```python
from build123d import *

# Parameters (mm, degrees)
F1_DEPTH = 10
F2_R     = 2.4
F3_DEPTH = 3
F7_R     = 5.08
F8_R     = 1.27


# Not quite as in the source:
# - a pattern or mirror of a feature is missing from the dataset's text; its kind, count and spacing are read off the source's solid


with BuildPart() as f1:
    # F0 (on Front) → F1 (new body)
    with BuildSketch(Plane.XZ):
        with BuildLine():
            ThreePointArc((0, 8.89), (6.2861792847, 6.2861792847), (8.89, 0))
            Line((8.89, 0), (8.89, -8.255))
            Line((8.89, -8.255), (21.89, -8.255))
            Line((21.89, -8.255), (21.89, -5.255))
            Line((21.89, -5.255), (11.89, -5.255))
            Line((11.89, -5.255), (11.89, 0))
            ThreePointArc((11.89, 0), (8.4074996283, 8.4074996283), (0, 11.89))
            Line((0, 11.89), (-5.255, 11.89))
            Line((-5.255, 11.89), (-5.255, 21.89))
            Line((-5.255, 21.89), (-8.255, 21.89))
            Line((-8.255, 21.89), (-8.255, 8.89))
            Line((-8.255, 8.89), (0, 8.89))
        make_face()
    extrude(amount=F1_DEPTH)

    # F2 (on face) → F3 (cut, through all)
    with BuildSketch(Plane.XY.offset(-5.255)):
        with Locations((16.89, -5)):
            Circle(F2_R)
    f3 = extrude(amount=-F3_DEPTH, mode=Mode.SUBTRACT)

    # F3_copies: F3 across plane
    add(f3.mirror(Plane(origin=(0, 0, 0), x_dir=(-0.7071067812, 0, -0.7071067812), z_dir=(-0.7071067812, 0, 0.7071067812))), mode=Mode.SUBTRACT)

    # F7
    f7_edges = [f1.edges().sort_by_distance(p)[0] for p in [
        (-8.255, -5, 8.89),
        (8.89, -5, -8.255),
    ]]
    fillet(f7_edges, radius=F7_R)

    # F8
    f8_edges = [f1.edges().sort_by_distance(p)[0] for p in [
        (-5.255, -5, 11.89),
        (11.89, -5, -5.255),
    ]]
    fillet(f8_edges, radius=F8_R)


solid = f1.part
```
Verification items for the finished model (mm, model axes). A direction names the side the tool comes from. Give positions to 0.01 mm unless a question says otherwise; leave off trailing zeros. Loops run counter-clockwise (first coordinate to the right, second up) from the corner with the lowest first, then second, coordinate; pieces in that order, holes last. Notation, with made-up numbers: M 40.25,71 L 48.25,71 A28 cw 48.25,107 Z; hole C -9.5,58 d4. An arc over 180 degrees is marked long. Return JSON: item names as keys, results as strings.
1) Section check D-D, the plane y = -1.5. Enter the section's corners in (x, z) (3 decimals), and give its area (3 significant figures).
Findings:
{"outline": "M -8.255,13.97 A5.08 ccw -3.175,8.89 L 0,8.89 A8.89 cw 8.89,0 L 8.89,-3.175 A5.08 ccw 13.97,-8.255 L 21.89,-8.255 L 21.89,-5.255 L 13.16,-5.255 A1.27 cw 11.89,-3.985 L 11.89,0 A11.89 ccw 0,11.89 L -3.985,11.89 A1.27 cw -5.255,13.16 L -5.255,21.89 L -8.255,21.89 Z", "area": "148 mm2"}
2) Mould release check, pull along Y, two halves, no side actions. Record for faces 1 (the flat face through (6, 0, 7)), 2 (the cylindrical face through (6.22, -4.93, 6.35)), 3 (the cylindrical face through (18.18, -2.976, -6.734)): released by +Y, released by -Y, zero draft, split by the parting line, or undercut.
Findings:
{"face 1": "released by +Y", "face 2": "zero draft", "face 3": "undercut"}
3) Section check A-A, the plane y = -5. Enter the section's corners in (x, z) (3 decimals), and give its area (3 significant figures).
Findings:
{"outline": "M -8.255,13.97 A5.08 ccw -3.175,8.89 L 0,8.89 A8.89 cw 8.89,0 L 8.89,-3.175 A5.08 ccw 13.97,-8.255 L 14.49,-8.255 L 14.49,-5.255 L 13.16,-5.255 A1.27 cw 11.89,-3.985 L 11.89,0 A11.89 ccw 0,11.89 L -3.985,11.89 A1.27 cw -5.255,13.16 L -5.255,14.49 L -8.255,14.49 Z; M -8.255,19.29 L -5.255,19.29 L -5.255,21.89 L -8.255,21.89 Z; M 19.29,-8.255 L 21.89,-8.255 L 21.89,-5.255 L 19.29,-5.255 Z", "area": "119 mm2"}
4) Section check C-C, the plane z = 16.89. Enter the section's corners in (x, y) (3 decimals), and give its area (3 significant figures).
Findings:
{"outline": "M -8.255,-10 L -5.255,-10 L -5.255,-7.4 L -8.255,-7.4 Z; M -8.255,-2.6 L -5.255,-2.6 L -5.255,0 L -8.255,0 Z", "area": "15.6 mm2"}
5) Material ranges on L1, parallel to X at y = -3, z = -1.5; L2, parallel to Z at x = 19.5, y = -8.25 (3 decimals), recorded low to high. Write a range as [from, to].
Findings:
{"L1": "x = [8.89, 11.89]", "L2": "z = [-8.255, -5.255]"}
6) Section check B-B, the plane x = 16.89. Enter the section's corners in (y, z) (3 decimals).
Findings:
{"outline": "M -10,-8.255 L -7.4,-8.255 L -7.4,-5.255 L -10,-5.255 Z; M -2.6,-8.255 L 0,-8.255 L 0,-5.255 L -2.6,-5.255 Z"}
7) Tool access check on faces 4 (the flat face through (8.89, -5, -2)), 5 (the flat face through (-8.255, -5, 20)), 6 (the flat face through (11.89, -5, -2)). Record the directions out of +Z, -Z, +X, -X, +Y, -Y that give a thin tool (end or side, any length) a straight path to the whole face; none if there is none.
Findings:
{"face 4": "-Z, -X, +Y, -Y", "face 5": "+Z, -Z, -X, +Y, -Y", "face 6": "+Z, +X, +Y, -Y"}
8) Gauge pin test, flat ends, axial feed: P1, Ø1.5, axis at x = 18.5, y = -6.5, coming from the +Z side (3 decimals); P2, Ø2.5, axis at x = -1, y = -4.5, coming from the -Z side; P3, Ø1.5, axis at x = 7, y = -3.5, coming from the -Z side. Record the tip position at first contact, or that the pin passes through.
Findings:
{"P1": "stops at z = -5.255", "P2": "stops at z = 8.89", "P3": "stops at z = 4.36"}
